Here's how the part is built. I have some questions about the finished solid (model axes, mm). Give positions to 0.01 mm unless a question says otherwise; leave off trailing zeros. Write each loop counter-clockwise with the first axis right and the second up, starting at its lowest first coordinate (ties: lowest second). Pieces come first, ordered by that corner, then holes. Notation, with made-up numbers: (-3.5, 49) - (47.5, 49) arc R16 ccw to (47.5, 71) - close; hole circle Ø10 at (51.25, 75.25). An arc over 180 degrees is marked (long way). One line per item, written item: value. Start each with the question number.
1) Imagine slicing it at A-A on y = -5. Write out the boundary of the cut face in (x, z).
2) Please list where these lines run through material, in increasing order: L1, parallel to Z at x = 7.25, y = -5; L2, parallel to X at y = -6.75, z = 21; L3, parallel to Z at x = 0.5, y = -4.5. Write a range as [from, to].
3) We'd pull the mould along Z, two halves only. Please class faces 1 (the flat face through (5, -5, 34)), 2 (the flat face through (5, -5, 0)), 3 (the cylindrical face through (5, -5, 24)), 4 (the flat face through (5, -10, 17)): +Z half, -Z half, draft (parallel to the pull), parting line (faces both ways), or undercut.
4) Imagine slicing it at B-B on x = 5. Write out the boundary of the cut face in (y, z).
5) I'm going to push a flat-ended pin straight in: P1, Ø3.5, axis at y = -5, z = 8, coming from the +X side. Where does the tip first touch, or does it pass through?
6) Imagine slicing it at D-D on x = 8.75. Write out the boundary of the cut face in (y, z), plus the area to 3 significant figures.
7) Imagine slicing it at C-C on z = 8. Write out the boundary of the cut face in (x, y).
from build123d import *

# Parameters (mm, degrees)
SKETCH_1_W          = 10
SKETCH_1_H          = 10
EXTRUDE_1_DEPTH     = 34
SKETCH_2_R          = 2
CUT_EXTRUDE_1_DEPTH = 37.823905279
SKETCH_3_R          = 2
CUT_EXTRUDE_2_DEPTH = 37.823905279


with BuildPart() as part:
    # 草图1 → 凸台-拉伸1 (new body)
    with BuildSketch(Plane.XY):
        with Locations((5, -5)):
            Rectangle(SKETCH_1_W, SKETCH_1_H)
    extrude(amount=EXTRUDE_1_DEPTH)

    # 草图2 → 切除-拉伸1 (cut, through all)
    with BuildSketch(Plane(origin=(10, 0, 0), x_dir=(0, 0, -1), z_dir=(1, 0, 0))):
        with Locations(Location((-26, -5, 0), (0, 0, 90))):
            Circle(SKETCH_2_R)
        with Locations(Location((-8, -5, 0), (0, 0, 90))):
            Circle(SKETCH_2_R)
    extrude(amount=-CUT_EXTRUDE_1_DEPTH, mode=Mode.SUBTRACT)

    # 草图3 → 切除-拉伸2 (cut, through all)
    with BuildSketch(Plane(origin=(0, 0, 0), x_dir=(1, 0, 0), z_dir=(0, 1, 0))):
        with Locations(Location((5, -13, 0), (0, 0, 270))):
            Circle(SKETCH_3_R)
        with Locations(Location((5, -21, 0), (0, 0, 270))):
            Circle(SKETCH_3_R)
    extrude(amount=-CUT_EXTRUDE_2_DEPTH, mode=Mode.SUBTRACT)


solid = part.part
Numbers:
1. outline: (0, 0) - (10, 0) - (10, 6) - (0, 6) - close; (0, 10) - (10, 10) - (10, 24) - (0, 24) - close; (0, 28) - (10, 28) - (10, 34) - (0, 34) - close; hole circle Ø4 at (5, 13); hole circle Ø4 at (5, 21)
2. L1: [0, 6], [10, 24], [28, 34]
2. L2: [0, 3], [7, 10]
2. L3: [0, 6.06], [9.94, 24.06], [27.94, 34]
3. face 1: +Z half
3. face 2: -Z half
3. face 3: undercut
3. face 4: draft
4. outline: (-10, 0) - (0, 0) - (0, 11) - (-10, 11) - close; (-10, 15) - (0, 15) - (0, 19) - (-10, 19) - close; (-10, 23) - (0, 23) - (0, 34) - (-10, 34) - close; hole circle Ø4 at (-5, 8); hole circle Ø4 at (-5, 26)
5. P1: through
6. outline: (-10, 0) - (0, 0) - (0, 34) - (-10, 34) - close; hole circle Ø4 at (-5, 8); hole circle Ø4 at (-5, 26)
6. area: 315 mm^2
7. outline: (0, -10) - (10, -10) - (10, -7) - (0, -7) - close; (0, -3) - (10, -3) - (10, 0) - (0, 0) - close
